Check sheet for the modelled part. Datum: model origin and axes. Units: mm. A direction names the side the tool comes from. Give positions to 0.01 mm unless a question says otherwise; leave off trailing zeros. Write each loop counter-clockwise with the first axis right and the second up, starting at its lowest first coordinate (ties: lowest second). Pieces come first, ordered by that corner, then holes. Notation, with made-up numbers: (-22, -26) - (28, -26) arc R21 cw to (28, -11) - close; hole circle Ø10 at (17.5, 39.25). An arc over 180 degrees is marked (long way). Return JSON: item names as keys, results as strings. Group by question number.
```python
from build123d import *

# Parameters (mm, degrees)
PROFILESKETCH1_W                = 100
PROFILESKETCH1_H                = 61
PROFILEBOSS_EXTRUDE1_DEPTH      = 25
CABLE_GUIDESSKETCH2_W           = 3
CABLE_GUIDESSKETCH2_H           = 61
CABLEGUIDESCUT_EXTRUDE1_DEPTH   = 23
FASTENERTABSKETCH1_W            = 10
FASTENERTABSKETCH1_H            = 39
FASTENERTABSKETCH1_H_2          = 61
FASTENERTABCUT_EXTRUDE1_DEPTH   = 23
FASTENINGHOLESKETCH2_R          = 1.5
FASTENINGHOLECUT_EXTRUDE2_DEPTH = 120.774788666
FILLET1_R                       = 3
FILLET2_R                       = 3


with BuildPart() as part:
    # ProfileSketch1 → ProfileBoss-Extrude1 (new body)
    with BuildSketch(Plane(origin=(0, 0, 0), x_dir=(1, 0, 0), z_dir=(0, 1, 0))):
        with Locations((50, 30.5)):
            Rectangle(PROFILESKETCH1_W, PROFILESKETCH1_H)
    extrude(amount=PROFILEBOSS_EXTRUDE1_DEPTH)

    # Cable GuidesSketch2 → CableGuidesCut-Extrude1 (cut)
    with BuildSketch(Plane(origin=(0, 25, 0), x_dir=(1, 0, 0), z_dir=(0, 1, 0))):
        Polygon((43.5, 61), (46.5, 61), (46.5, 2), (0, 2), (0, 5), (43.5, 5), align=None)
        Polygon((0, 20), (0, 17), (16.5, 17), (16.5, 61), (13.5, 61), (13.5, 20), align=None)
        Polygon((0, 7), (36.5, 7), (36.5, 61), (33.5, 61), (33.5, 10), (0, 10), align=None)
        Polygon((0, 12), (26.5, 12), (26.5, 61), (23.5, 61), (23.5, 15), (0, 15), align=None)
        with Locations((55, 30.5)):
            Rectangle(CABLE_GUIDESSKETCH2_W, CABLE_GUIDESSKETCH2_H)
        with Locations((65, 30.5)):
            Rectangle(CABLE_GUIDESSKETCH2_W, CABLE_GUIDESSKETCH2_H)
        with Locations((75, 30.5)):
            Rectangle(CABLE_GUIDESSKETCH2_W, CABLE_GUIDESSKETCH2_H)
        with Locations((85, 30.5)):
            Rectangle(CABLE_GUIDESSKETCH2_W, CABLE_GUIDESSKETCH2_H)
    extrude(amount=-CABLEGUIDESCUT_EXTRUDE1_DEPTH, mode=Mode.SUBTRACT)

    # FastenerTabSketch1 → FastenerTabCut-Extrude1 (cut)
    with BuildSketch(Plane(origin=(0, 25, 0), x_dir=(1, 0, 0), z_dir=(0, 1, 0))):
        with Locations((5, 41.5)):
            Rectangle(FASTENERTABSKETCH1_W, FASTENERTABSKETCH1_H)
        with Locations((95, 30.5)):
            Rectangle(FASTENERTABSKETCH1_W, FASTENERTABSKETCH1_H_2)
    extrude(amount=-FASTENERTABCUT_EXTRUDE1_DEPTH, mode=Mode.SUBTRACT)

    # FasteningHoleSketch2 → FasteningHoleCut-Extrude2 (cut, through all)
    with BuildSketch(Plane(origin=(0, 25, 0), x_dir=(1, 0, 0), z_dir=(0, 1, 0))):
        with Locations(Location((6.5, 31, 0), (0, 0, 270))):
            Circle(FASTENINGHOLESKETCH2_R)
        with Locations(Location((93.5, 31, 0), (0, 0, 270))):
            Circle(FASTENINGHOLESKETCH2_R)
    extrude(amount=-FASTENINGHOLECUT_EXTRUDE2_DEPTH, mode=Mode.SUBTRACT)

    # Fillet1
    fillet1_edges = [part.edges().sort_by_distance(p)[0] for p in [
        (43.5, 13.5, -5),
        (23.5, 13.5, -15),
        (33.5, 13.5, -10),
        (13.5, 13.5, -20),
    ]]
    fillet(fillet1_edges, radius=FILLET1_R)

    # Fillet2
    fillet2_edges = [part.edges().sort_by_distance(p)[0] for p in [
        (46.5, 13.5, -2),
        (10, 13.5, -22),
        (26.5, 13.5, -12),
        (36.5, 13.5, -7),
        (16.5, 13.5, -17),
    ]]
    fillet(fillet2_edges, radius=FILLET2_R)


solid = part.part
```
Item 1: Section check B-B on x = 29. Record the cut outline in (y, z), plus the area to 3 significant figures.
Item 2: Section check C-C on z = -31. Count the separate pieces of the cut face and the enclosed holes in it, plus the area to 3 significant figures.
Item 3: Material ranges on line 1 along Z through (x, y) = (27.5, 17.75); line 2 along X through (y, z) = (1.5, -31); line 3 along Z through (x, y) = (18, 14.5), recorded low to high. Write a range as from..to.
Item 4: Mould release check, pull along X, two halves, no side actions. Record for faces 4 (the face through (63.5, 14, -30)), 5 (the face through (0, 8.7, -16.8)), 6 (the face through (11, 25, -39)): +X half, -X half, draft (parallel to the pull), parting line (faces both ways), or undercut.
Item 5: Depth check by flat-ended pin: pin 1 (1.5 mm diameter, centred on x = 75.5, z = -23, fed in from +Y); pin 2 (7 mm diameter, centred on y = 10.5, z = -38.5, fed in from +X); pin 3 (5 mm diameter, centred on y = 11.5, z = -36.5, fed in from -X). Enter the tip coordinate at first touch or a pass-through.
Item 6: Section check A-A on x = 93.5. Record the cut outline in (y, z), plus the area to 3 significant figures.
Item 7: Access from +Z, -Z, +X, -X, +Y, -Y to the whole of each face (thin tool, end or side, straight path). Record for faces 1 (the face through (73.5, 14, -30)), 2 (the face through (15.64, 13.34, -17.9)), 3 (the face through (96, 2, -31)).
Reply:
{
 "1": {"outline": "(0, -61) - (25, -61) - (25, -10) - (2, -10) - (2, -7) - (25, -7) - (25, -5) - (2, -5) - (2, -2) - (25, -2) - (25, 0) - (0, 0) - close", "area": "1,390 mm²"},
 "2": {"separate pieces": "3", "enclosed holes": "0", "area": "1,480 mm²"},
 "3": {"line 1": "-61..-10, -7..-5, -2..0", "line 2": "0..5, 8..92, 95..100", "line 3": "-61..-15, -12..-10, -7..-5, -2..0"},
 "4": {"face 4": "undercut", "face 5": "-X half", "face 6": "draft"},
 "5": {"pin 1": "y = 2", "pin 2": "x = 90", "pin 3": "x = 10"},
 "6": {"outline": "(0, -61) - (2, -61) - (2, -32.5) - (0, -32.5) - close; (0, -29.5) - (2, -29.5) - (2, 0) - (0, 0) - close", "area": "116 mm²"},
 "7": {"face 1": "+Z, -Z, +Y", "face 2": "-Z, -X, +Y", "face 3": "+Z, -Z, +X, +Y"}
}
